Geometry check sheet. Reference: drawing and pictorial views, mm from the part's lowest x, y, z. A direction names the side the tool comes from. Round coordinates to 2 decimals unless told otherwise and drop trailing zeros. Write each loop counter-clockwise with the first axis right and the second up, starting at its lowest first coordinate (ties: lowest second). Pieces come first, ordered by that corner, then holes. Notation, with made-up numbers: (22.25, -23.75) - (39.25, -23.75) arc R16 cw to (39.25, -19.75) - close; hole circle Ø6 at (25.25, 27.25). An arc over 180 degrees is marked (long way). Use one line per item in the form item = value. Start each with the question number.
1) Section check A-A (z = 81.2). Record the boundary of the cut face in (x, y).
2) Draft check along Y on the marked faces 3, 4 and 5. Enter one of: +Y half, -Y half, draft (parallel to the pull), parting line (faces both ways), or undercut.
3) Scan lines: probe 1 along Y at (x, z) = (325, 80); probe 2 along Z at (x, y) = (323, 70.5); probe 3 along X at (y, z) = (98.5, 53) (1 decimal). Record each from-to range of solid material in increasing order.
4) Section check B-B (z = 214.76). Record the boundary of the cut face in (x, y).
5) Section check D-D (y = 14). Record the boundary of the cut face in (x, z).
6) Set-up check for the marked faces 1 and 2: record each of +Z, -Z, +X, -X, +Y, -Y from which the full face is reachable in a straight line by a thin tool's end or side.
7) Section check C-C (x = 276). Record the boundary of the cut face in (y, z) (1 decimal), then the cut area to 3 significant figures.
8) Gauge pin test, flat ends, axial feed: P1, Ø3, axis at x = 123, y = 105.5, coming from the +Z side; P2, Ø5, axis at x = 176.5, z = 56.5, coming from the -Y side; P3, Ø5, axis at x = 357.5, z = 97.5, coming from the +Y side. Record the tip position at first contact, or that the pin passes through.
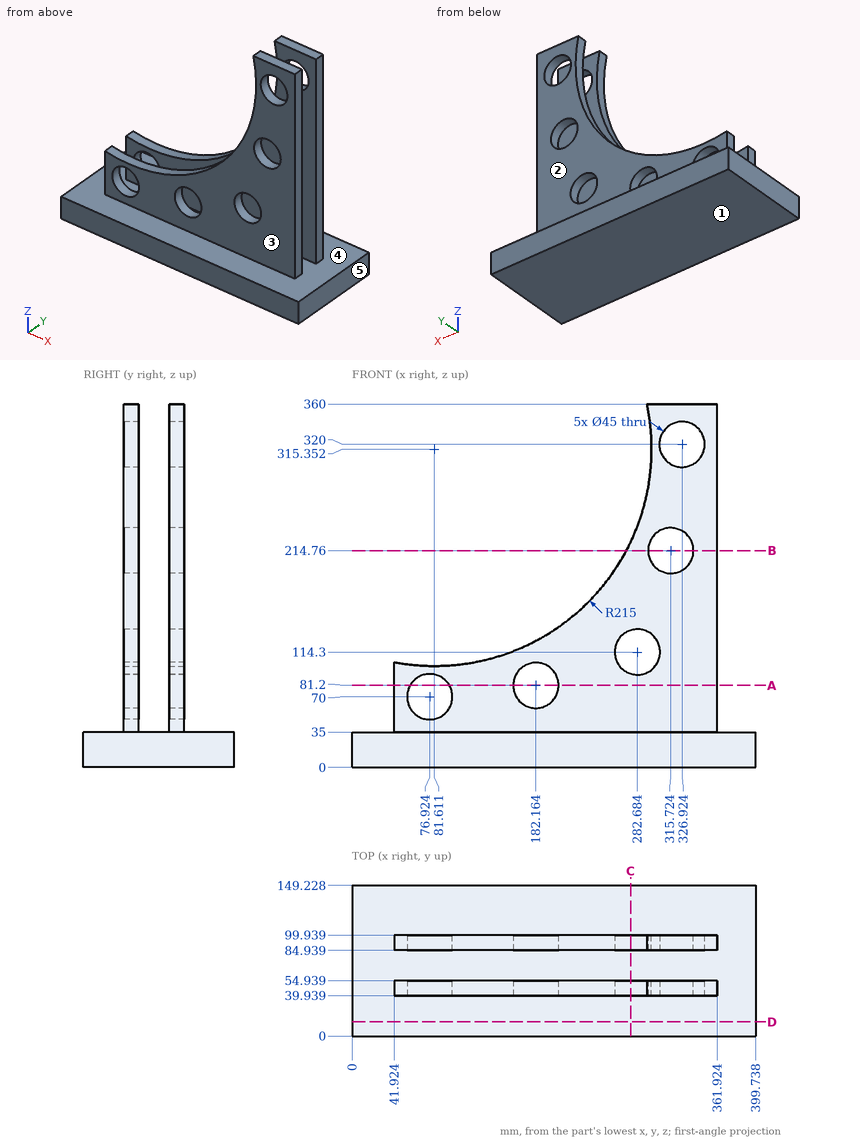
Results are:
q1.outline = (41.92, 39.94) - (57.41, 39.94) - (57.41, 54.94) - (41.92, 54.94) - close; (41.92, 84.94) - (57.41, 84.94) - (57.41, 99.94) - (41.92, 99.94) - close; (96.44, 39.94) - (159.66, 39.94) - (159.66, 54.94) - (96.44, 54.94) - close; (96.44, 84.94) - (159.66, 84.94) - (159.66, 99.94) - (96.44, 99.94) - close; (204.66, 39.94) - (361.92, 39.94) - (361.92, 54.94) - (204.66, 54.94) - close; (204.66, 84.94) - (361.92, 84.94) - (361.92, 99.94) - (204.66, 99.94) - close
q2.face_3 = -Y half
q2.face_4 = undercut
q2.face_5 = draft
q3.probe_1 = 39.94 to 54.94, 84.94 to 99.94
q3.probe_2 = 0 to 35
q3.probe_3 = 41.9 to 62.2, 91.7 to 361.9
q4.outline = (271.63, 39.94) - (293.22, 39.94) - (293.22, 54.94) - (271.63, 54.94) - close; (271.63, 84.94) - (293.22, 84.94) - (293.22, 99.94) - (271.63, 99.94) - close; (338.22, 39.94) - (361.92, 39.94) - (361.92, 54.94) - (338.22, 54.94) - close; (338.22, 84.94) - (361.92, 84.94) - (361.92, 99.94) - (338.22, 99.94) - close
q5.outline = (0, 0) - (399.74, 0) - (399.74, 35) - (0, 35) - close
q6.face_1 = -Z, +X, -X, +Y, -Y
q6.face_2 = +Z, +X, -X, +Y
q7.outline = (0, 0) - (149.2, 0) - (149.2, 35) - (99.9, 35) - (99.9, 92.8) - (84.9, 92.8) - (84.9, 35) - (54.9, 35) - (54.9, 92.8) - (39.9, 92.8) - (39.9, 35) - (0, 35) - close; (39.9, 135.8) - (54.9, 135.8) - (54.9, 223.5) - (39.9, 223.5) - close; (84.9, 135.8) - (99.9, 135.8) - (99.9, 223.5) - (84.9, 223.5) - close
q7.area = 9,590 mm²
q8.P1 = 35
q8.P2 = 39.94
q8.P3 = 99.94
